Geometry: final body of the model. Coordinates: model frame, mm. Face numbers are marked on the shaded views. Give positions to 0.01 mm unless a question says otherwise; leave off trailing zeros. Loops run counter-clockwise (first coordinate to the right, second up) from the corner with the lowest first, then second, coordinate; pieces in that order, holes last. Notation, with made-up numbers: (75, -12) - (99, -12) arc R27 cw to (99, 26) - close; hole circle Ø9 at (-15.5, 45.25). An arc over 180 degrees is marked (long way). Answer in a Markdown table with one row per item.
from build123d import *

# Parameters (mm, degrees)
F1_ANGLE = 170
F2_SIZE  = 0.5
F3_R     = 2
F4_SIZE  = 0.5


# Not quite as in the source:
# - a feature names something its author has since deleted; it is built from what else it names


with BuildPart() as f1:
    # F0 (on Front) → F1 (revolve)
    with BuildSketch(Plane.XZ):
        Polygon((-48.5, 9), (-48.5, 0), (-46.5, 0), (-46.5, 8), (-42.5, 8), (-38.5, 7.5), (-36.5, 7.5), (-36.5, 9), align=None)
    revolve(axis=Axis((0, 0, 4.2486875318), (0, 0, 1)), revolution_arc=F1_ANGLE)

    # F2
    f2_edges = [f1.edges().sort_by_distance(p)[0] for p in [
        (-4.052742, -46.323053, 0),
    ]]
    chamfer(f2_edges, length=F2_SIZE)

    # F3
    f3_edges = [f1.edges().sort_by_distance(p)[0] for p in [
        (47.02457, -8.2917, 0),
        (-47.75, 0, 0),
    ]]
    fillet(f3_edges, radius=F3_R)

    # F4
    f4_edges = [f1.edges().sort_by_distance(p)[0] for p in [
        (-3.181185, -36.361106, 9),
    ]]
    chamfer(f4_edges, length=F4_SIZE)


solid = f1.part
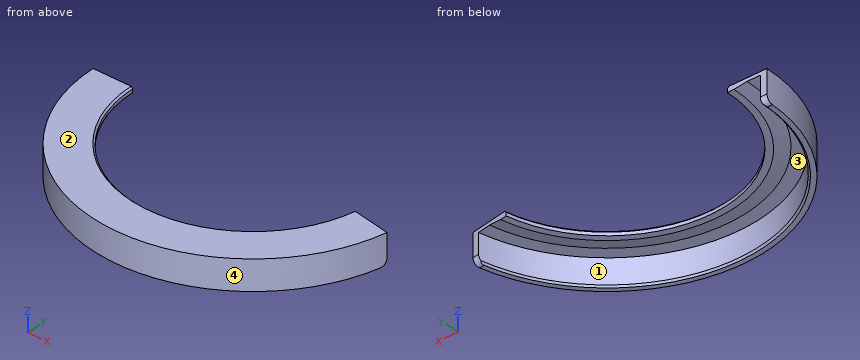
Q1. Cut plane A-A (z = 6.5). Output: boundary loops of the cut face in (x, y), and give its area (3 significant figures).
Check values:
| item | result |
|---|---|
| outline | (-48.5, 0) arc R48.5 ccw to (47.76, -8.42) - (45.79, -8.07) arc R46.5 cw to (-46.5, 0) - close |
| area | 282 mm² |
Q2. Draft query along X for the marked faces 1, 2, 3 and 4. Return one class per face: pulls with the +X half, pulls with the -X half, needs draft (parallel to the pull), parting line crosses it, or undercut.
Check values:
| item | result |
|---|---|
| face 1 | undercut |
| face 2 | needs draft |
| face 3 | undercut |
| face 4 | parting line crosses it |
Q3. Material intervals for line 1 along Y through (x, z) = (-1, 2); line 2 along X through (y, z) = (-31.5, 5.25); line 3 along X through (y, z) = (-22.5, 2.75), sorted ascending.
Check values:
| item | result |
|---|---|
| line 1 | -48.49 to -46.49 |
| line 2 | -36.88 to -34.21, 34.21 to 36.88 |
| line 3 | -42.97 to -40.69, 40.69 to 42.97 |
Q4. First-contact query: pin 1 (4 mm diameter, centred on y = -22, z = 2, fed in from +X); pin 2 (2 mm diameter, centred on y = -16.5, z = 5.5, fed in from -X); pin 3 (2 mm diameter, centred on x = 16, z = 1.5, fed in from +Y). Flat tips, straight axial feed; report the tip coordinate or a pass-through.
Check values:
| item | result |
|---|---|
| pin 1 | x = 44.18 |
| pin 2 | x = -45.96 |
| pin 3 | y = -43.28 |
